Design review of the part built by this model. Coordinates are the model's own, in mm. A direction names the side the tool comes from. Coordinates: 2 decimals unless noted, no trailing zeros. Write each loop counter-clockwise with the first axis right and the second up, starting at its lowest first coordinate (ties: lowest second). Pieces come first, ordered by that corner, then holes. Notation, with made-up numbers: (40.25, -37) - (76.25, -37) arc R16 cw to (76.25, -6) - close; hole circle Ø5 at (73, -15). An arc over 180 degrees is marked (long way). Answer as a JSON object with one key per item and string values.
```python
from build123d import *

# Parameters (mm, degrees)
F0_W     = 1.74625
F0_H     = 5.15
F0_W_2   = 5
F0_H_2   = 1.5875
F1_DEPTH = 1.5875
F2_R     = 5


# Not quite as in the source:
# - a length typed as a fraction of an inch, garbled in the dataset ("3 / 203.2 mm" for 3/8 in), is restored


with BuildPart() as f1:
    # F0 (on Right) → F1 (new body)
    with BuildSketch(Plane.YZ):
        with BuildLine():
            Line((20, -15), (20, 15))
            Line((20, 15), (8.075, 15))
            ThreePointArc((8.075, 15), (0, 6.925), (-8.075, 15))
            Line((-8.075, 15), (-20, 15))
            Line((-20, 15), (-20, -15))
            Line((-20, -15), (-17.5, -15))
            Line((-17.5, -15), (-12.5, -15))
            Line((-12.5, -15), (-10, -15))
            Line((-10, -15), (-10, -5))
            Line((-10, -5), (10, -5))
            Line((10, -5), (10, -15))
            Line((10, -15), (12.5, -15))
            Line((12.5, -15), (17.5, -15))
            Line((17.5, -15), (20, -15))
        make_face()
        with Locations((-14.6303550991, -10)):
            Rectangle(F0_W, F0_H, mode=Mode.SUBTRACT)
        with Locations((15.5080378336, -10)):
            Rectangle(F0_W, F0_H, mode=Mode.SUBTRACT)
        with Locations((-15, 10)):
            Rectangle(F0_W, F0_H, mode=Mode.SUBTRACT)
        with Locations((15, 10)):
            Rectangle(F0_W, F0_H, mode=Mode.SUBTRACT)
        with Locations((-15, -15.79375)):
            Rectangle(F0_W_2, F0_H_2)
        with Locations((15, -15.79375)):
            Rectangle(F0_W_2, F0_H_2)
    extrude(amount=F1_DEPTH)

    # F2
    f2_edges = [f1.edges().sort_by_distance(p)[0] for p in [
        (0.79375, -10, -5),
        (0.79375, 10, -5),
        (0.79375, 20, 15),
        (0.79375, -20, 15),
    ]]
    fillet(f2_edges, radius=F2_R)


solid = f1.part
```
(1) The part is to be moulded in two halves that separate along Y. For faces 1 (the face through (1, -13.757, -10)), 2 (the face through (1, -17.5, -16)), 3 (the face through (1.588, 0, -1)), say which applies: pulls with the +Y half, pulls with the -Y half, needs draft (parallel to the pull), parting line crosses it, or undercut.
Solved:
{"face 1": "undercut", "face 2": "pulls with the -Y half", "face 3": "needs draft"}
(2) Take a section at A-A, the plane z = -6. Write out the cut boundary in (x, y), and give its area (3 significant figures).
Solved:
{"outline": "(0, -20) - (1.59, -20) - (1.59, -8) - (0, -8) - close; (0, 8) - (1.59, 8) - (1.59, 20) - (0, 20) - close", "area": "38.1 mm^2"}
(3) To check wall thickness, follow line 1 (Y direction, x = 1.15, z = -13); line 2 (Z direction, x = 0.65, y = 14.5) (1 decimal); line 3 (Z direction, x = 0.5, y = -12). State the ranges of each line that lie inside material, in increasing order. Write a range as from..to.
Solved:
{"line 1": "y = -20..-10, 10..20", "line 2": "z = -16.6..7.4, 12.6..15", "line 3": "z = -15..15"}
(4) Tool access review of faces 4 (the face through (1, -15.873, 10)), 5 (the face through (1, 19, -15)), 6 (the face through (1, -12.5, -16)): name each direction out of +Z, -Z, +X, -X, +Y, -Y from which nothing blocks a thin tool from reaching the whole face with its end or side.
Solved:
{"face 4": "+X, -X", "face 5": "-Z, +X, -X, +Y", "face 6": "-Z, +X, -X"}
(5) Take a section at B-B, the plane x = 0.95. Give the number of separate pieces and of enclosed holes in the cut face, and give its area (3 significant figures).
Solved:
{"separate pieces": "1", "enclosed holes": "4", "area": "877 mm^2"}
(6) Take a section at D-D, the plane z = 13. Write out the cut boundary in (x, y), and give its area (3 significant figures).
Solved:
{"outline": "(0, -19) - (1.59, -19) - (1.59, -7.82) - (0, -7.82) - close; (0, 7.82) - (1.59, 7.82) - (1.59, 19) - (0, 19) - close", "area": "35.5 mm^2"}
(7) Take a section at C-C, the plane y = 0. Write out the cut boundary in (x, z) (1 decimal).
Solved:
{"outline": "(0, -5) - (1.6, -5) - (1.6, 6.9) - (0, 6.9) - close"}
(8) For pin 1 (0.5 mm diameter, centred on x = 1, z = -15.5, fed in from -Y); pin 2 (0.8 mm diameter, centred on x = 1, y = 1, fed in from -Z); pin 3 (0.8 mm diameter, centred on x = 1, y = -18.5, fed in from -Z), all flat-tipped, find the tip position at first contact; note any pin that passes through.
Solved:
{"pin 1": "stops at y = -17.5", "pin 2": "stops at z = -5", "pin 3": "stops at z = -15"}
